Autodesk Inventor part; units mm, degrees
ref_plane "YZ Plane" through (0, 0, 0) normal (1, 0, 0) x (0, 1, 0)
ref_plane "XZ Plane" through (0, 0, 0) normal (0, 1, 0) x (-1, 0, 0)
ref_plane "XY Plane" through (0, 0, 0) normal (0, 0, 1) x (1, 0, 0)
sketch "Sketch1" plane through (0, 0, 0) normal (0, 0, 1) x (1, 0, 0)
  line L0 (0, 2.8582) -> (0, -2.8582) construction
  line L1 (-5.7775, 0) -> (5.7775, 0) construction
  line L2 (-165, -75) -> (165, -75)
  line L3 (165, -75) -> (165, 75)
  line L4 (165, 75) -> (-165, 75)
  line L5 (-165, 75) -> (-165, -75)
  line L6 (-165, -75) -> (165, 75) construction
  line L7 (165, -75) -> (-165, 75) construction
  point P0 (0, 0)
  point P1 (0, 0)
  dimension "d0" = 330
  dimension "d1" = 150
extrude "Extrusion1" add sketch "Sketch1" along normal blind 5
sketch "Sketch2" plane through (0, 0, 5) normal (0, 0, 1) x (1, 0, 0)
  line L0 (0, 0) -> (-130, 0)
  circle A0 centre (-130, 0) radius 5
  line L1 (-165, 75) -> (-165, -75)
  line L2 (-165, 0) -> (-165, 15)
  line L3 (-165, 15) -> (-165, -15)
  line L4 (-165, -15) -> (-165, -45)
  line L5 (-165, -45) -> (-165, -75)
  line L6 (-165, 15) -> (-165, 45)
  line L7 (-165, 45) -> (-165, 75)
  line L8 (-165, 15) -> (-160, 15)
  line L9 (-160, 15) -> (-160, 45)
  line L10 (-160, 45) -> (-165, 45)
  line L11 (-165, 45) -> (-165, 15)
  line L12 (-165, -15) -> (-160, -15)
  line L13 (-160, -15) -> (-160, -45)
  line L14 (-160, -45) -> (-165, -45)
  line L15 (-165, -45) -> (-165, -15)
  line L16 (-165, -75) -> (165, -75)
  line L17 (-165, -75) -> (-135, -75)
  line L18 (-135, -75) -> (-105, -75)
  line L19 (-105, -75) -> (-75, -75)
  line L20 (-75, -75) -> (-45, -75)
  line L21 (-45, -75) -> (-15, -75)
  line L22 (-15, -75) -> (15, -75)
  line L23 (15, -75) -> (45, -75)
  line L24 (45, -75) -> (75, -75)
  line L25 (75, -75) -> (105, -75)
  line L26 (105, -75) -> (135, -75)
  line L27 (135, -75) -> (165, -75)
  line L28 (-165, -75) -> (-135, -75)
  line L29 (-135, -75) -> (-135, -70)
  line L30 (-135, -70) -> (-165, -70)
  line L31 (-165, -70) -> (-165, -75)
  line L32 (-105, -75) -> (-75, -75)
  line L33 (-75, -75) -> (-75, -70)
  line L34 (-75, -70) -> (-105, -70)
  line L35 (-105, -70) -> (-105, -75)
  line L36 (-45, -75) -> (-15, -75)
  line L37 (-15, -75) -> (-15, -70)
  line L38 (-15, -70) -> (-45, -70)
  line L39 (-45, -70) -> (-45, -75)
  line L40 (15, -75) -> (45, -75)
  line L41 (45, -75) -> (45, -70)
  line L42 (45, -70) -> (15, -70)
  line L43 (15, -70) -> (15, -75)
  line L44 (75, -75) -> (105, -75)
  line L45 (105, -75) -> (105, -70)
  line L46 (105, -70) -> (75, -70)
  line L47 (75, -70) -> (75, -75)
  line L48 (135, -75) -> (165, -75)
  line L49 (165, -75) -> (165, -70)
  line L50 (165, -70) -> (135, -70)
  line L51 (135, -70) -> (135, -75)
  line L52 (165, 75) -> (-165, 75)
  line L53 (-165, 75) -> (-135, 75)
  line L54 (-135, 75) -> (-135, 70)
  line L55 (-135, 70) -> (-165, 70)
  line L56 (-165, 70) -> (-165, 75)
  line L57 (-105, 75) -> (-75, 75)
  line L58 (-75, 75) -> (-75, 70)
  line L59 (-75, 70) -> (-105, 70)
  line L60 (-105, 70) -> (-105, 75)
  line L61 (-45, 75) -> (-15, 75)
  line L62 (-15, 75) -> (-15, 70)
  line L63 (-15, 70) -> (-45, 70)
  line L64 (-45, 70) -> (-45, 75)
  line L65 (15, 75) -> (45, 75)
  line L66 (45, 75) -> (45, 70)
  line L67 (45, 70) -> (15, 70)
  line L68 (15, 70) -> (15, 75)
  line L69 (75, 75) -> (105, 75)
  line L70 (105, 75) -> (105, 70)
  line L71 (105, 70) -> (75, 70)
  line L72 (75, 70) -> (75, 75)
  line L73 (165, -75) -> (165, 75)
  line L74 (135, 75) -> (165, 75)
  line L75 (165, 75) -> (165, 70)
  line L76 (165, 70) -> (135, 70)
  line L77 (135, 70) -> (135, 75)
  line L78 (165, 0) -> (165, 15)
  line L79 (165, 15) -> (160, 15)
  line L80 (160, 15) -> (160, 45)
  line L81 (160, 45) -> (165, 45)
  line L82 (165, 45) -> (165, 15)
  line L83 (165, -15) -> (160, -15)
  line L84 (160, -15) -> (160, -45)
  line L85 (160, -45) -> (165, -45)
  line L86 (165, -45) -> (165, -15)
  point P0 (-165, -70)
  point P1 (135, 75)
  point P2 (105, 75)
  point P3 (75, 75)
  point P4 (45, 75)
  point P5 (15, 75)
  point P6 (-15, 75)
  point P7 (-165, 70)
  point P8 (-165, -45)
  dimension "d4" = 130
  dimension "d5" = 10
  dimension "d6" = 15
  dimension "d7" = 30
  dimension "d8" = 30
  dimension "d9" = 30
  dimension "d10" = 30
  dimension "d11" = 30
  dimension "d12" = 5
  dimension "d13" = 30
  dimension "d14" = 30
  dimension "d15" = 30
  dimension "d16" = 30
  dimension "d17" = 30
  dimension "d18" = 30
  dimension "d19" = 30
  dimension "d20" = 30
  dimension "d21" = 30
  dimension "d22" = 30
  dimension "d23" = 30
  dimension "d24" = 5
  dimension "d25" = 5
  dimension "d26" = 5
  dimension "d29" = 30
  dimension "d30" = 30
  dimension "d31" = 30
  dimension "d32" = 30
  dimension "d33" = 30
  dimension "d34" = 30
extrude "Extrusion2" cut sketch "Sketch2" against normal blind 8 contours A0 | L52 L54 L55 L1 | L10 L9 L8 L1 | L52 L58 L59 L60 | L52 L62 L63 L64 | L12 L13 L14 L1 | L52 L66 L67 L68 | L30 L29 L16 L1 | L52 L70 L71 L72 | L35 L34 L33 L16 | L52 L73 L76 L77 | L39 L38 L37 L16 | L73 L79 L80 L81 | L43 L42 L41 L16 | L47 L46 L45 L16 | L73 L85 L84 L83 | L51 L50 L49 L16
sketch "Sketch3" plane through (0, 0, 5) normal (0, 0, 1) x (1, 0, 0)
  line L0 (165, -15) -> (165, 15)
  line L1 (165, 0) -> (85, 0)
  circle A0 centre (85, 0) radius 33.5
  point P0 (0, 0)
  dimension "d35" = 80
  dimension "d36" = 67
extrude "Extrusion3" cut sketch "Sketch3" against normal blind 10
sketch "Sketch4" plane through (0, 0, 5) normal (0, 0, 1) x (1, 0, 0)
  circle A0 centre (85, 0) radius 33.5
  line L0 (85, 0) -> (85, 42)
  circle A1 centre (85, 42) radius 2.5
  line L1 (85, 0) -> (85, -42)
  circle A2 centre (85, -42) radius 2.5
  point P0 (0, 0)
  dimension "d39" = 42
  dimension "d40" = 5
  dimension "d41" = 42
  dimension "d42" = 5
extrude "Extrusion4" cut sketch "Sketch4" against normal blind 5 contours A2 | A1
sketch "Sketch5" plane through (0, 0, 5) normal (0, 0, 1) x (1, 0, 0)
  line L0 (165, -70) -> (135, -70)
  line L1 (165, -70) -> (-75, -70)
  line L2 (-75, -75) -> (-45, -75)
  line L3 (-75, -75) -> (-184.16, -75)
  line L4 (-184.16, -75) -> (-184.16, 77.2339)
  line L5 (-184.16, 77.2339) -> (-75, 77.2339)
  line L6 (-75, 77.2339) -> (-75, -75)
  point P0 (0, 0)
  dimension "d45" = 240
extrude "Extrusion5" cut sketch "Sketch5" against normal blind 5
sketch "Sketch6" plane through (0, 0, 5) normal (0, 0, 1) x (1, 0, 0)
  line L0 (-75, 75) -> (-75, -75)
  line L1 (-75, 0) -> (-55, 0)
  line L2 (-55, 0) -> (-52, 0)
  line L3 (-55, -8) -> (-52, -8)
  line L4 (-52, -8) -> (-52, 8)
  line L5 (-52, 8) -> (-55, 8)
  line L6 (-55, 8) -> (-55, -8)
  line L7 (-55, -8) -> (-52, 8) construction
  line L8 (-52, -8) -> (-55, 8) construction
  point P0 (0, 0)
  point P1 (-53.5, 0)
  dimension "d25" = 5
  dimension "d48" = 20
  dimension "d49" = 3
  dimension "d50" = 3
  dimension "d51" = 16
extrude "Extrusion6" cut sketch "Sketch6" against normal blind 10
properties part number "Plaat boven" material "S235"
Source: CAD feature listing. Evaluate the final solid. Frame: model axes, mm. A direction names the side the tool comes from. Round coordinates to 2 decimals unless told otherwise and drop trailing zeros. Loops run counter-clockwise (first coordinate to the right, second up) from the corner with the lowest first, then second, coordinate; pieces in that order, holes last. Notation, with made-up numbers: M 33.25,65 L 83.25,65 A26 cw 83.25,88 Z; hole C 19.25,16 d9. An arc over 180 degrees is marked long. Use a Markdown table: item, result. Add a question column.
1. Cut plane A-A, the plane y = 0. Output: boundary loops of the cut face in (x, z).
2. Ray query, line 1 along Y through (x, z) = (85, 3.15); line 2 along X through (y, z) = (42, 4.05); line 3 along X through (y, z) = (2, 0.4). Return the intervals inside material, ascending. Write a range as [from, to].
3. Pull-direction query (Y, two-part tool) for faces 1 (the flat face through (135, 72, 3)), 2 (the flat face through (120, 75, 2)), 3 (the flat face through (162, 45, 3)); classes: +Y half, -Y half, draft (parallel to the pull), parting line (faces both ways), or undercut.
4. Cut plane D-D, the plane z = 2.9. State how many separate pieces and enclosed holes the cut face has, and give its area (3 significant figures).
5. Cut plane C-C, the plane y = -42. Output: boundary loops of the cut face in (x, z), and give its area (3 significant figures).
6. Set-up query: faces 4 (the flat face through (162, -45, 3)), 5 (the flat face through (-45, 72, 3)), 6 (the flat face through (0, -75, 2)), 7 (the flat face through (135, -72, 3)), 8 (the flat face through (60, 75, 2)). Return all of +Z, -Z, +X, -X, +Y, -Y with unobstructed straight access to the full face (end or side cutting, diameter ignored); none if empty.
7. Cut plane B-B, the plane x = 85. Output: boundary loops of the cut face in (y, z).
8. Contact query for flat-ended pins moving along their axis: pin 1 (2.5 mm diameter, centred on x = 86, z = 1.5, fed in from +Y); pin 2 (1.5 mm diameter, centred on x = 86, z = 2, fed in from -Y); pin 3 (2.5 mm diameter, centred on y = 71.5, z = 2, fed in from +X); pin 4 (10 mm diameter, centred on x = -15.5, y = 58, fed in from -Z). Output: stop coordinate, or through.
Solution:
| question | item | result |
|---|---|---|
| 1 | outline | M -75,0 L -55,0 L -55,5 L -75,5 Z; M -52,0 L 51.5,0 L 51.5,5 L -52,5 Z; M 118.5,0 L 165,0 L 165,5 L 118.5,5 Z |
| 2 | line 1 | y = [-70, -44.5], [-39.5, -33.5], [33.5, 39.5], [44.5, 70] |
| 2 | line 2 | x = [-75, 82.5], [87.5, 160] |
| 2 | line 3 | x = [-75, -55], [-52, 51.56], [118.44, 165] |
| 3 | face 1 | draft |
| 3 | face 2 | +Y half |
| 3 | face 3 | undercut |
| 4 | separate pieces | 1 |
| 4 | enclosed holes | 4 |
| 4 | area | 30,900 mm2 |
| 5 | outline | M -75,0 L 82.5,0 L 82.5,5 L -75,5 Z; M 87.5,0 L 160,0 L 160,5 L 87.5,5 Z |
| 5 | area | 1,150 mm2 |
| 6 | face 4 | +Z, -Z, +X |
| 6 | face 5 | +Z, -Z, +Y |
| 6 | face 6 | +Z, -Z, +X, -X, -Y |
| 6 | face 7 | +Z, -Z, +X, -Y |
| 6 | face 8 | +Z, -Z, +X, -X, +Y |
| 7 | outline | M -70,0 L -44.5,0 L -44.5,5 L -70,5 Z; M -39.5,0 L -33.5,0 L -33.5,5 L -39.5,5 Z; M 33.5,0 L 39.5,0 L 39.5,5 L 33.5,5 Z; M 44.5,0 L 70,0 L 70,5 L 44.5,5 Z |
| 8 | pin 1 | stops at y = 70 |
| 8 | pin 2 | stops at y = -70 |
| 8 | pin 3 | stops at x = 135 |
| 8 | pin 4 | stops at z = 0 |
